Can you work these out from the model? Positions are in its coordinate system, mm. A direction names the side the tool comes from. Give positions to 0.01 mm unless a question says otherwise; leave off trailing zeros. Order: outer loops, then holes, each group sorted by start corner. A loop starts at its lowest first (then second) coordinate and runs counter-clockwise, first axis right, second up.
Item 1: I'm going to push flat-ended pins straight in: pin 1 Ø1.5 at (y, z) = (-11.5, 323.5) entering from -X; pin 2 Ø7.5 at (x, y) = (-685.5, -16) entering from +Z. Where does each tip first touch, or does it pass through?
Item 2: I want a section at C-C, the plane x = -669.5. Write out the boundary of the cut face in (y, z), then the cut area to 3 significant figures.
Item 3: I want a section at B-B, the plane z = 329. Write out the boundary of the cut face in (x, y).
Item 4: Which directions (+Z, -Z, +X, -X, +Y, -Y) give clear straight access to the entire face, cutting with the end or side of a thin tool? Please do faces 1 (the flat face through (-386, -12, 0)), 2 (the flat face through (-635, -12, 318)).
Item 5: I want a section at A-A, the plane y = -11.25. Write out the boundary of the cut face in (x, z), then the cut area to 3 significant figures.
Item 6: If I drill on line 1 along Z through (x, y) = (-102, -5.5); line 2 along Z through (x, y) = (-678, -3); line 3 along X through (y, z) = (-15, 342.5), over which ranges is the centre line in solid material (lowest first)?
```python
from build123d import *

# Parameters (mm, degrees)
F1_DEPTH = 25
F2_R     = 6
F3_R     = 6


with BuildPart() as f1:
    # F0 (on Front) → F1 (new body)
    with BuildSketch(Plane.XZ):
        Polygon((0, 381), (-635, 381), (-635, 254), (-762, 254), (-762, 0), (0, 0), align=None)
    extrude(amount=F1_DEPTH)

    # F2
    f2_edges = [f1.edges().sort_by_distance(p)[0] for p in [
        (-317.5, -25, 381),
    ]]
    fillet(f2_edges, radius=F2_R)

    # F3
    f3_edges = [f1.edges().sort_by_distance(p)[0] for p in [
        (-317.5, 0, 381),
    ]]
    fillet(f3_edges, radius=F3_R)


solid = f1.part
```
Results list:
1. pin 1: stops at x = -635
1. pin 2: stops at z = 254
2. outline: (-25, 0) - (0, 0) - (0, 254) - (-25, 254) - close
2. area: 6,350 mm2
3. outline: (-635, -25) - (0, -25) - (0, 0) - (-635, 0) - close
4. face 1: -Z, +X, -X, +Y, -Y
4. face 2: +Z, -X, +Y, -Y
5. outline: (-762, 0) - (0, 0) - (0, 381) - (-635, 381) - (-635, 254) - (-762, 254) - close
5. area: 274,000 mm2
6. line 1: z = 0 to 380.98
6. line 2: z = 0 to 254
6. line 3: x = -635 to 0
